CAD build for the part. Positions are in the model's coordinates, mm. A direction names the side the tool comes from. Give positions to 0.01 mm unless a question says otherwise; leave off trailing zeros. Loops run counter-clockwise (first coordinate to the right, second up) from the corner with the lowest first, then second, coordinate; pieces in that order, holes last.
Item 1: Drop flat-ended pins along their axis: P1, Ø3.5, axis at x = 0, z = 27.5, coming from the +Y side; P2, Ø1, axis at x = -0.5, z = 18.5, coming from the +Y side; P3, Ø12, axis at y = 7, z = 2.5, coming from the -X side. Give the stop position or say it passes through.
Item 2: Saw through at A-A on z = 0. Give the cut face in (x, y).
Item 3: Probe probe 1 along Z at (x, y) = (0.5, -3); probe 2 along Z at (x, y) = (-1.5, -3.25); probe 3 along Y at (x, z) = (-1.5, -7). List the from-to ranges inside material, lowest first.
Item 4: Saw through at B-B on z = -12. Give the cut face in (x, y), plus the area to 3 significant figures.
Item 5: Saw through at C-C on y = -7.75. Give the cut face in (x, z), plus the area to 3 significant figures.
Item 6: Which spindle directions (+Z, -Z, +X, -X, +Y, -Y) get a long thin tool onto all of the face, cutting with end or side? Do faces 1 (the cylindrical face through (-0.608, 10.195, 14.895)), 2 (the flat face through (0, 7.77, 30)), 3 (the flat face through (-1, 9, 7.5)), 4 (the flat face through (0, 7.77, -30)). Say none if no direction does.
Item 7: Mould opens along Z. For faces 5 (the flat face through (-2, -1, -1)), 6 (the flat face through (-1, 9, -7.5)), 7 (the flat face through (-1, 9, 22.5)) say: released by +Z, released by -Z, zero draft, split by the parting line, or undercut.
Item 8: Saw through at D-D on z = -27.5. Give the cut face in (x, y).
from build123d import *

# Parameters (mm, degrees)
BOSS_EXTRUDE1_DEPTH      = 37.5
BOSS_EXTRUDE1_DEPTH_BACK = 37.5
SKETCH1_R                = 1.5
CUT_EXTRUDE1_DEPTH       = 37.5
CUT_EXTRUDE1_DEPTH_BACK  = 37.5
SKETCH2_R                = 1.5
SKETCH2_W                = 15
SKETCH2_H                = 15


with BuildPart() as part:
    # Sketch1 → Boss-Extrude1 (new, two sides: drawn at the far end of the back side and taken through both)
    with BuildSketch(Plane.XY.offset(-BOSS_EXTRUDE1_DEPTH_BACK)):
        with BuildLine():
            Line((-2, 7.769691362), (-2, -9.423076923))
            Line((-2, -9.423076923), (1, -9.423076923))
            Line((1, -9.423076923), (1, 10.576923077))
            ThreePointArc((1, 10.576923077), (-4.043575876, 12.960215003), (-2, 7.769691362))
        make_face()
        with Locations((-1.993800738, 10.769684957)):
            Circle(SKETCH1_R, mode=Mode.SUBTRACT)
    extrude(amount=BOSS_EXTRUDE1_DEPTH + BOSS_EXTRUDE1_DEPTH_BACK)

    # Sketch2 → Cut-Extrude1 (cut, two sides: drawn at the far end of the back side and taken through both)
    with BuildSketch(Plane.ZY.offset(2).offset(-CUT_EXTRUDE1_DEPTH_BACK)):
        with Locations(Location((-22.5, -3.423076923, 0), (0, 0, 180))):
            Circle(SKETCH2_R)
        with Locations(Location((0, -3.423076923, 0), (0, 0, 180))):
            Circle(SKETCH2_R)
        with Locations(Location((22.5, -3.423076923, 0), (0, 0, 180))):
            Circle(SKETCH2_R)
        with Locations((-30, 15.269691362)):
            Rectangle(SKETCH2_W, SKETCH2_H)
        with Locations((0, 15.269691362)):
            Rectangle(SKETCH2_W, SKETCH2_H)
        with Locations((30, 15.269691362)):
            Rectangle(SKETCH2_W, SKETCH2_H)
    extrude(amount=CUT_EXTRUDE1_DEPTH + CUT_EXTRUDE1_DEPTH_BACK, mode=Mode.SUBTRACT)


solid = part.part
Results below:
1. P1: stops at y = 7.77
1. P2: stops at y = 13.6
1. P3: stops at x = -4.96
2. outline: (-2, -9.42) - (1, -9.42) - (1, -4.92) - (-2, -4.92) - close; (-2, -1.92) - (1, -1.92) - (1, 7.77) - (-2, 7.77) - close
3. probe 1: z = -37.5 to -23.94, -21.06 to -1.44, 1.44 to 21.06, 23.94 to 37.5
3. probe 2: z = -37.5 to -23.99, -21.01 to -1.49, 1.49 to 21.01, 23.99 to 37.5
3. probe 3: y = -9.42 to 7.77
4. outline: (-2, -9.42) - (1, -9.42) - (1, 10.58) arc R3 ccw (long way) to (-2, 7.77) - close; hole circle Ø3 at (-1.99, 10.77)
4. area: 74.7 mm2
5. outline: (-2, -37.5) - (1, -37.5) - (1, 37.5) - (-2, 37.5) - close
5. area: 225 mm2
6. face 1: +Z, -Z
6. face 2: +Z, +X, -X, +Y
6. face 3: +X, -X, +Y
6. face 4: -Z, +X, -X, +Y
7. face 5: zero draft
7. face 6: undercut
7. face 7: released by +Z
8. outline: (-2, -9.42) - (1, -9.42) - (1, 7.77) - (-2, 7.77) - close
